Geometry check sheet. Reference: the model listing, model coordinates, mm. A direction names the side the tool comes from. Give positions to 0.01 mm unless a question says otherwise; leave off trailing zeros. Loops run counter-clockwise (first coordinate to the right, second up) from the corner with the lowest first, then second, coordinate; pieces in that order, holes last. Notation, with made-up numbers: (4, -7.5) -> (51, -7.5) arc R27 ccw to (51, 9.5) -> close; hole circle Ø11 at (74.5, 62.5). An arc over 180 degrees is marked (long way). Write item = value, one per line.
```python
from build123d import *

# Parameters (mm, degrees)
RESSALTO_EXTRUS_O1_DEPTH      = 2
FILETE1_R                     = 10
RESSALTO_EXTRUS_O2_DEPTH      = 2
RESSALTO_EXTRUS_O2_DEPTH_BACK = 4
CORTE_EXTRUS_O1_DEPTH         = 106
ESBO_O5_R                     = 32.5
CORTE_EXTRUS_O2_DEPTH         = 106


with BuildPart() as part:
    # Esboço1 → Ressalto-extrusão1 (new body)
    with BuildSketch(Plane(origin=(0, 0, 0), x_dir=(1, 0, 0), z_dir=(0, 1, 0))):
        Polygon((0, 0), (100.1, 0), (100.1, 130.2), (42.5645027, 90), align=None)
    extrude(amount=RESSALTO_EXTRUS_O1_DEPTH)

    # Filete1
    filete1_edges = [part.edges().sort_by_distance(p)[0] for p in [
        (42.5645027, 1, -90),
    ]]
    fillet(filete1_edges, radius=FILETE1_R)

    # Esboço2 → Ressalto-extrusão2 (add, two sides: drawn at the far end of the back side and taken through both)
    with BuildSketch(Plane(origin=(0, 0, 0), x_dir=(-1, 0, 0), z_dir=(0, -1, 0)).offset(-RESSALTO_EXTRUS_O2_DEPTH_BACK)):
        Polygon((-100.1, 0), (-100.1, 7.845993173), (-3.710675529, 7.845993173), (0, 0), align=None)
    extrude(amount=RESSALTO_EXTRUS_O2_DEPTH + RESSALTO_EXTRUS_O2_DEPTH_BACK)

    # Esboço4 → Corte-extrusão1 (cut)
    with BuildSketch(Plane(origin=(100.1, 0, 0), x_dir=(0, 0, -1), z_dir=(1, 0, 0))):
        with BuildLine():
            Line((0, 4), (7.845993173, 4))
            Line((7.845993173, 4), (7.845993173, 2))
            add(Edge.make_bspline(
                [(7.845993173, 2), (3.140345255, 1.903943557), (0, 4)],
                knots=[0, 0, 0, 1, 1, 1], degree=2))
        make_face()
        with BuildLine():
            Line((7.845993173, 0), (7.845993173, -2))
            Line((7.845993173, -2), (0, -2))
            add(Edge.make_bspline(
                [(7.845993173, 0), (3.106908611, 0.009053077), (0, -2)],
                knots=[0, 0, 0, 1, 1, 1], degree=2))
        make_face()
    extrude(amount=-CORTE_EXTRUS_O1_DEPTH, mode=Mode.SUBTRACT)

    # Esboço5 → Corte-extrusão2 (cut)
    with BuildSketch(Plane(origin=(100.1, 0, 0), x_dir=(0, 0, -1), z_dir=(1, 0, 0))):
        with Locations((-32, 0.73240575)):
            Circle(ESBO_O5_R)
    extrude(amount=-CORTE_EXTRUS_O2_DEPTH, mode=Mode.SUBTRACT)


solid = part.part
```
Item 1: Gauge pin test, flat ends, axial feed: pin 1 (12 mm diameter, centred on x = 55, z = -83, fed in from +Y); pin 2 (1 mm diameter, centred on y = 1.5, z = -100.5, fed in from -X); pin 3 (1 mm diameter, centred on x = 73.5, z = -96, fed in from -Y). Record the tip position at first contact, or that the pin passes through.
Answer:
pin_1 = 2
pin_2 = 56.88
pin_3 = 0
Item 2: Section check A-A, the plane z = -90. Record the cut outline in (x, y).
Answer:
outline = (43.02, 0) -> (100.1, 0) -> (100.1, 2) -> (43.02, 2) -> close
Item 3: Thickness scan on L1, parallel to Y at x = 84, z = -57; L2, parallel to X at y = 0.5, z = -7; L3, parallel to Z at x = 87.5, y = 3. Record the ranges inside material, lowest first. Write a range as [from, to].
Answer:
L1 = [0, 2]
L2 = [3.31, 100.1]
L3 = [-1.88, -0.42]
Item 4: Tool access check on faces 1 (the flat face through (100.1, 1, -65)), 2 (the flat face through (62, 2, -56)), 3 (the flat face through (62, 0, -56)). Record the directions out of +Z, -Z, +X, -X, +Y, -Y that give a thin tool (end or side, any length) a straight path to the whole face; none if there is none.
Answer:
face_1 = +Z, -Z, +X, +Y, -Y
face_2 = -Z, +X, -X, +Y
face_3 = -Z, +X, -X, -Y
Item 5: Section check B-B, the plane z = -42. Record the cut outline in (x, y), plus the area to 3 significant figures.
Answer:
outline = (19.86, 0) -> (100.1, 0) -> (100.1, 2) -> (19.86, 2) -> close
area = 160 mm^2
